Build history of the part. All positions in model axes, mm. Face numbers are marked on the shaded views. Give positions to 0.01 mm unless a question says otherwise; leave off trailing zeros. Loops run counter-clockwise (first coordinate to the right, second up) from the corner with the lowest first, then second, coordinate; pieces in that order, holes last. Notation, with made-up numbers: (69.25, 55) - (97.25, 55) arc R33 ccw to (97.25, 92) - close; hole circle Ø3 at (32.5, 65.25). An arc over 180 degrees is marked (long way). Return JSON: item names as keys, results as strings. Group by question number.
1) Drill centre lines: probe 1 along X at (y, z) = (-15.5, 6.75); probe 2 along Z at (x, y) = (-6.5, -4); probe 3 along Y at (x, z) = (-4, 10). Where is each one in solid material? Low to high. Write a range as from..to.
2) Drop flat-ended pins along their axis: pin 1 (6 mm diameter, centred on y = -14.5, z = 8, fed in from -X); pin 2 (14 mm diameter, centred on x = 6.5, y = -1, fed in from +Z); pin 3 (3 mm diameter, centred on x = 13, z = 1.5, fed in from -Y). Give the stop position or say it passes through.
3) Slice it at B-B (z = 6.5). List the corners of the cut face in (x, y), and give its area (3 significant figures).
4) Slice it at A-A (x = 0). List the corners of the cut face in (y, z), and give its area (3 significant figures).
5) Mould opens along X. For the marked faces 1, 2, 3 and 4 say: released by +X, released by -X, zero draft, split by the parting line, or undercut.
```python
from build123d import *

# Parameters (mm, degrees)
F1_DEPTH = 12
F2_R     = 3
F3_R     = 2
F5_DEPTH = 3
F6_R     = 3
F7_R     = 1
F8_R     = 1


with BuildPart() as f1:
    # F0 (on Top) → F1 (new body)
    with BuildSketch(Plane.XY):
        Polygon((10.9696551146, 19), (-10.9696551146, 19), (-21.9393102292, 0), (-10.9696551146, -19), (10.9696551146, -19), (21.9393102292, 0), align=None)
    extrude(amount=F1_DEPTH)

    # F2
    f2_edges = [f1.edges().sort_by_distance(p)[0] for p in [
        (-10.969655, -19, 6),
        (10.969655, -19, 6),
        (21.93931, 0, 6),
        (-21.93931, 0, 6),
        (-10.969655, 19, 6),
        (10.969655, 19, 6),
    ]]
    fillet(f2_edges, radius=F2_R)

    # F3
    f3_edges = [f1.edges().sort_by_distance(p)[0] for p in [
        (16.454483, 9.5, 0),
        (21.475209, 0, 0),
        (10.737604, 18.598076, 0),
        (16.454483, -9.5, 0),
        (0, 19, 0),
        (10.737604, -18.598076, 0),
        (-10.737604, 18.598076, 0),
        (0, -19, 0),
        (-16.454483, 9.5, 0),
        (-10.737604, -18.598076, 0),
        (-21.475209, 0, 0),
        (-16.454483, -9.5, 0),
    ]]
    fillet(f3_edges, radius=F3_R)

    # F4 (on face) → F5 (cut)
    with BuildSketch(Plane.XY.offset(12)):
        Polygon((8.6602540378, 15), (-8.6602540378, 15), (-17.3205080757, 0), (-8.6602540378, -15), (8.6602540378, -15), (17.3205080757, 0), align=None)
    extrude(amount=-F5_DEPTH, mode=Mode.SUBTRACT)

    # F6
    f6_edges = [f1.edges().sort_by_distance(p)[0] for p in [
        (-8.660254, 15, 10.5),
        (8.660254, 15, 10.5),
        (17.320508, 0, 10.5),
        (-17.320508, 0, 10.5),
        (-8.660254, -15, 10.5),
        (8.660254, -15, 10.5),
    ]]
    fillet(f6_edges, radius=F6_R)

    # F7
    f7_edges = [f1.edges().sort_by_distance(p)[0] for p in [
        (0, 15, 12),
        (8.428203, 14.598076, 12),
        (-8.428203, 14.598076, 12),
        (12.990381, 7.5, 12),
        (-12.990381, 7.5, 12),
        (16.856406, 0, 12),
        (-16.856406, 0, 12),
        (12.990381, -7.5, 12),
        (-12.990381, -7.5, 12),
        (8.428203, -14.598076, 12),
        (-8.428203, -14.598076, 12),
        (0, -15, 12),
        (16.454483, 9.5, 12),
        (21.475209, 0, 12),
        (10.737604, 18.598076, 12),
        (16.454483, -9.5, 12),
        (0, 19, 12),
        (10.737604, -18.598076, 12),
        (-10.737604, 18.598076, 12),
        (0, -19, 12),
        (-16.454483, 9.5, 12),
        (-10.737604, -18.598076, 12),
        (-21.475209, 0, 12),
        (-16.454483, -9.5, 12),
    ]]
    fillet(f7_edges, radius=F7_R)

    # F8
    f8_edges = [f1.edges().sort_by_distance(p)[0] for p in [
        (0, 15, 9),
        (8.428203, 14.598076, 9),
        (-8.428203, 14.598076, 9),
        (12.990381, 7.5, 9),
        (-12.990381, 7.5, 9),
        (16.856406, 0, 9),
        (-16.856406, 0, 9),
        (12.990381, -7.5, 9),
        (-12.990381, -7.5, 9),
        (8.428203, -14.598076, 9),
        (-8.428203, -14.598076, 9),
        (0, -15, 9),
    ]]
    fillet(f8_edges, radius=F8_R)


solid = f1.part
```
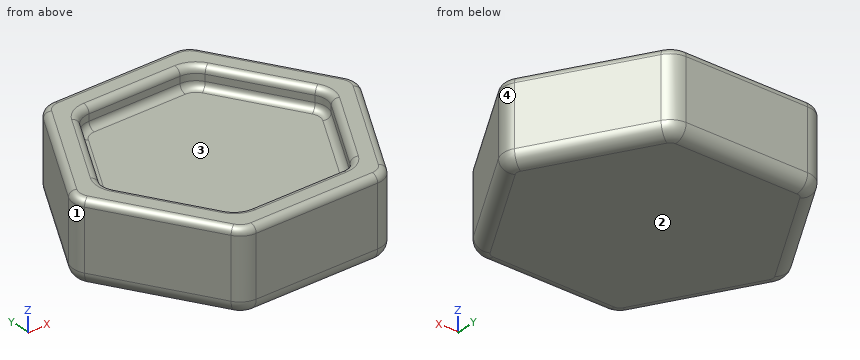
Results:
{
 "1": {"probe 1": "-12.99..12.99", "probe 2": "0..9", "probe 3": "-19..-15, 15..19"},
 "2": {"pin 1": "x = -15.3", "pin 2": "z = 9", "pin 3": "y = -17.92"},
 "3": {"outline": "(-21.07, -1.5) - (-11.84, -17.5) arc R3 ccw to (-9.24, -19) - (9.24, -19) arc R3 ccw to (11.84, -17.5) - (21.07, -1.5) arc R3 ccw to (21.07, 1.5) - (11.84, 17.5) arc R3 ccw to (9.24, 19) - (-9.24, 19) arc R3 ccw to (-11.84, 17.5) - (-21.07, 1.5) arc R3 ccw to start", "area": "1,250 mm2"},
 "4": {"outline": "(-19, 2) arc R2 ccw to (-17, 0) - (17, 0) arc R2 ccw to (19, 2) - (19, 11) arc R1 ccw to (18, 12) - (16, 12) arc R1 ccw to (15, 11) - (15, 10) arc R1 cw to (14, 9) - (-14, 9) arc R1 cw to (-15, 10) - (-15, 11) arc R1 ccw to (-16, 12) - (-18, 12) arc R1 ccw to (-19, 11) - close", "area": "364 mm2"},
 "5": {"face 1": "released by -X", "face 2": "zero draft", "face 3": "undercut", "face 4": "released by +X"}
}
